from build123d import *

# Parameters (mm, degrees)
SKETCH1_W               = 240
SKETCH1_H               = 240
BOSS_EXTRUDE1_DEPTH     = 15
SKETCH3_R               = 15
BOSS_EXTRUDE3_DEPTH     = 250
MIRROR7_COPY_1_SKETCH_R = 15
MIRROR7_COPY_1_DEPTH    = 250
SKETCH4_R               = 10.5
CUT_EXTRUDE1_DEPTH      = 250
SKETCH5_R               = 1.15
CUT_EXTRUDE2_DEPTH      = 40
MIRROR9_COPY_1_SKETCH_R = 1.15
MIRROR9_COPY_1_DEPTH    = 40
SKETCH6_R               = 5
CUT_EXTRUDE3_DEPTH      = 30


with BuildPart() as part:
    # Sketch1 → Boss-Extrude1 (new body)
    with BuildSketch(Plane.XY):
        Rectangle(SKETCH1_W, SKETCH1_H)
    extrude(amount=BOSS_EXTRUDE1_DEPTH)

    # Sketch3 → Boss-Extrude3 (add)
    with BuildSketch(Plane(origin=(0, 0, 0), x_dir=(-1, 0, 0), z_dir=(0, 0, -1))):
        with Locations((90, -90)):
            Circle(SKETCH3_R)
    boss_extrude3 = extrude(amount=BOSS_EXTRUDE3_DEPTH)

    # Mirror6: Boss-Extrude3 across plane
    add(boss_extrude3.mirror(Plane.ZX))

    # Mirror7: Boss-Extrude3 across plane
    add(boss_extrude3.mirror(Plane(origin=(0, 0, 0), x_dir=(0, 0, 1), z_dir=(1, 0, 0))))

    # Mirror7 copy 1 sketch → Mirror7 copy 1 (add)
    with BuildSketch(Plane(origin=(0, 0, 0), x_dir=(1, 0, 0), z_dir=(0, 0, -1))):
        with Locations((90, -90)):
            Circle(MIRROR7_COPY_1_SKETCH_R)
    extrude(amount=MIRROR7_COPY_1_DEPTH)

    # Sketch4 → Cut-Extrude1 (cut)
    with BuildSketch(Plane.XY.offset(15)):
        Circle(SKETCH4_R)
    extrude(amount=-CUT_EXTRUDE1_DEPTH, mode=Mode.SUBTRACT)

    # Sketch5 → Cut-Extrude2 (cut)
    with BuildSketch(Plane.XY.offset(15)):
        with Locations((37.455598714, 21.625)):
            Circle(SKETCH5_R)
        with Locations((49.146941665, 28.375)):
            Circle(SKETCH5_R)
        with Locations((0, 43.25)):
            Circle(SKETCH5_R)
        with Locations((0, 56.75)):
            Circle(SKETCH5_R)
    cut_extrude2 = extrude(amount=-CUT_EXTRUDE2_DEPTH, mode=Mode.SUBTRACT)

    # Mirror8: Cut-Extrude2 across plane
    add(cut_extrude2.mirror(Plane.ZX), mode=Mode.SUBTRACT)

    # Mirror9: Cut-Extrude2 across plane
    add(cut_extrude2.mirror(Plane(origin=(0, 0, 0), x_dir=(0, 0, 1), z_dir=(1, 0, 0))), mode=Mode.SUBTRACT)

    # Mirror9 copy 1 sketch → Mirror9 copy 1 (cut)
    with BuildSketch(Plane(origin=(0, 0, 15), x_dir=(-1, 0, 0), z_dir=(0, 0, 1))):
        with Locations((37.455598714, 21.625)):
            Circle(MIRROR9_COPY_1_SKETCH_R)
        with Locations((49.146941665, 28.375)):
            Circle(MIRROR9_COPY_1_SKETCH_R)
        with Locations((0, 43.25)):
            Circle(MIRROR9_COPY_1_SKETCH_R)
        with Locations((0, 56.75)):
            Circle(MIRROR9_COPY_1_SKETCH_R)
    extrude(amount=-MIRROR9_COPY_1_DEPTH, mode=Mode.SUBTRACT)

    # Sketch6 → Cut-Extrude3 (cut)
    with BuildSketch(Plane.XY.offset(15)):
        with Locations((0, -110.68)):
            Circle(SKETCH6_R)
        with Locations((-95.851691691, 55.34)):
            Circle(SKETCH6_R)
        with Locations((95.851691691, 55.34)):
            Circle(SKETCH6_R)
    extrude(amount=-CUT_EXTRUDE3_DEPTH, mode=Mode.SUBTRACT)


solid = part.part
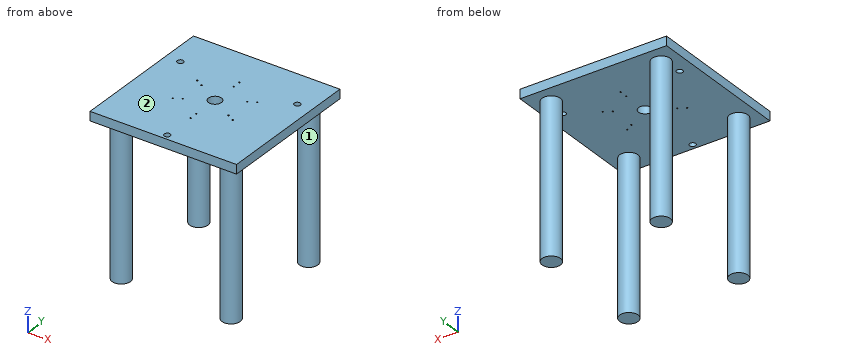
The model under review builds one solid part; all positions refer to its coordinate system, in mm. Face numbers are marked on the shaded views. Round coordinates to 2 decimals unless told otherwise and drop trailing zeros. Write each loop counter-clockwise with the first axis right and the second up, starting at its lowest first coordinate (ties: lowest second). Pieces come first, ordered by that corner, then holes. Notation, with made-up numbers: (66.25, 12) - (78.25, 12) arc R19 cw to (78.25, 24) - close; hole circle Ø4 at (4, 66). An arc over 180 degrees is marked (long way). One line per item, written item: value. Start each with the question number.
1. Clearance check with flat-ended pins moving along their axes: P1, Ø1.5, axis at x = -3.5, y = 14, coming from the -Z side; P2, Ø4, axis at y = -79, z = -93.5, coming from the -X side. State where each tip first meets the part, or that it passes through.
2. Consider section B-B on z = -84. Write out the cut boundary in (x, y).
3. To check wall thickness, follow L1, parallel to X at y = 43, z = 3; L2, parallel to Z at x = -101.5, y = -60; L3, parallel to X at y = 81, z = -18. State the ranges of each line that lie inside material, in increasing order. Write a range as from..to.
4. The part is to be moulded in two halves that separate along Y. For the marked faces 1 and 2, say which applies: released by +Y, released by -Y, zero draft, split by the parting line, or undercut.
5. Consider section D-D on x = 42.5. Write out the cut boundary in (y, z), and give its area (3 significant figures).
6. Consider section A-A on y = 0. Write out the cut boundary in (x, z), and give its area (4 significant figures).
7. Consider section C-C on y = 90. Write out the cut boundary in (x, z).
Checks:
1. P1: stops at z = 0
1. P2: stops at x = -102
2. outline: circle Ø30 at (-90, -90); circle Ø30 at (-90, 90); circle Ø30 at (90, -90); circle Ø30 at (90, 90)
3. L1: x = -120..-1.12, 1.12..120
3. L2: z = 0..15
3. L3: x = -102..-78, 78..102
4. face 1: undercut
4. face 2: zero draft
5. outline: (-120, 0) - (120, 0) - (120, 15) - (-120, 15) - close
5. area: 3,600 mm^2
6. outline: (-120, 0) - (-10.5, 0) - (-10.5, 15) - (-120, 15) - close; (10.5, 0) - (120, 0) - (120, 15) - (10.5, 15) - close
6. area: 3,285 mm^2
7. outline: (-120, 0) - (-105, 0) - (-105, -250) - (-75, -250) - (-75, 0) - (75, 0) - (75, -250) - (105, -250) - (105, 0) - (120, 0) - (120, 15) - (-120, 15) - close
